Verification items for the finished model (mm, model axes). A direction names the side the tool comes from. Round coordinates to 2 decimals unless told otherwise and drop trailing zeros. Order: outer loops, then holes, each group sorted by start corner. A loop starts at its lowest first (then second) coordinate and runs counter-clockwise, first axis right, second up. Notation, with made-up numbers: M 40.25,-1.5 L 58.25,-1.5 A10 ccw 58.25,11.5 Z; hole C 65.25,59 d6. An arc over 180 degrees is marked long. Use one line per item in the form item = value. Start each with the question number.
Item 1: Thickness scan on probe 1 along X at (y, z) = (22, -120.65); probe 2 along Y at (x, z) = (1.5, -72.5); probe 3 along Z at (x, y) = (-11.5, -7) (3 decimals). Record the ranges inside material, lowest first. Write a range as [from, to].
Item 2: Cross-section at C-C on y = 0. Enter the section's corners in (x, z) (3 decimals), then the cut area to 3 significant figures.
Item 3: Cross-section at B-B on z = -120.65. Enter the section's corners in (x, y), then the cut area to 3 significant figures.
Item 4: Cross-section at A-A on x = -12.7. Enter the section's corners in (y, z) (3 decimals), then the cut area to 3 significant figures.
Item 5: Go/stop test with flat-tipped pins: pin 1 Ø3 at (x, y) = (-15.88, 21.82) entering from +Z; pin 2 Ø2.5 at (x, y) = (9.19, 9.19) entering from +Z (3 decimals); pin 3 Ø12 at (x, y) = (-14, 0.5) entering from -Z; pin 4 Ø2 at (x, z) = (10.5, -63.5) entering from -Y. Record where each tip stops, or that it passes through.
Item 6: Release check for a two-part mould opening along Z. For faces 4 (the cylindrical face through (12.881, 21.863, -119.273)), 5 (the cylindrical face through (12.881, 21.863, -20.848)), 6 (the cylindrical face through (-14.91, 23.32, 1.57)), 7 (the flat face through (0, 11, 3.175)) record: +Z half, -Z half, draft (parallel to the pull), parting line (faces both ways), or undercut.
Item 7: Cross-section at D-D on x = 0. Enter the section's corners in (y, z) (3 decimals), then the cut area to 3 significant figures.
Item 8: Tool access check on faces 1 (the cylindrical face through (-0.23, 23.59, 1.57)), 2 (the flat face through (0, 24.994, -61)), 3 (the flat face through (-0.3, 10.2, 0)). Record the directions out of +Z, -Z, +X, -X, +Y, -Y that give a thin tool (end or side, any length) a straight path to the whole face; none if there is none.
from build123d import *

# Parameters (mm, degrees)
SKETCH1_W           = 38.1
SKETCH1_H           = 37.6936
SKETCH1_R           = 10
SKETCH1_R_2         = 1.5
SKETCH1_R_3         = 1.7859375
BOSS_EXTRUDE1_DEPTH = 3.175
SKETCH2_W           = 38.1
SKETCH2_H           = 6.35
BOSS_EXTRUDE2_DEPTH = 127
CUT_EXTRUDE1_REACH  = 135.838
SKETCH3_R           = 1.3890625


with BuildPart() as part:
    # Sketch1 → Boss-Extrude1 (new body)
    with BuildSketch(Plane.XY):
        with Locations((0, 6.1468)):
            Rectangle(SKETCH1_W, SKETCH1_H)
        Circle(SKETCH1_R, mode=Mode.SUBTRACT)
        with Locations((-9.192388155, 9.192388155)):
            Circle(SKETCH1_R_2, mode=Mode.SUBTRACT)
        with Locations((9.192388155, 9.192388155)):
            Circle(SKETCH1_R_2, mode=Mode.SUBTRACT)
        with Locations((9.192388155, -9.192388155)):
            Circle(SKETCH1_R_2, mode=Mode.SUBTRACT)
        with Locations((-9.192388155, -9.192388155)):
            Circle(SKETCH1_R_2, mode=Mode.SUBTRACT)
        with Locations((15.875, 21.8186)):
            Circle(SKETCH1_R_3, mode=Mode.SUBTRACT)
        with Locations((0, 21.8186)):
            Circle(SKETCH1_R_3, mode=Mode.SUBTRACT)
        with Locations((-15.875, 21.8186)):
            Circle(SKETCH1_R_3, mode=Mode.SUBTRACT)
    extrude(amount=BOSS_EXTRUDE1_DEPTH)

    # Sketch2 → Boss-Extrude2 (add)
    with BuildSketch(Plane(origin=(0, 0, 0), x_dir=(-1, 0, 0), z_dir=(0, 0, -1))):
        with Locations((0, 21.8186)):
            Rectangle(SKETCH2_W, SKETCH2_H)
    extrude(amount=BOSS_EXTRUDE2_DEPTH)

    # Sketch3 → Cut-Extrude1 (cut, up to next)
    with BuildSketch(Plane(origin=(0, 24.9936, 0), x_dir=(1, 0, 0), z_dir=(0, 1, 0)), mode=Mode.PRIVATE) as cut_extrude1_sk1:
        with Locations(Location((-12.7, 120.65, 0), (0, 0, 180))):
            Circle(SKETCH3_R)
    cut_extrude1_tool1 = extrude(cut_extrude1_sk1.sketch, amount=-CUT_EXTRUDE1_REACH, mode=Mode.PRIVATE) & part.part
    # Sketch3 → Cut-Extrude1 (cut, up to next)
    with BuildSketch(Plane(origin=(0, 24.9936, 0), x_dir=(1, 0, 0), z_dir=(0, 1, 0)), mode=Mode.PRIVATE) as cut_extrude1_sk2:
        with Locations(Location((12.7, 120.65, 0), (0, 0, 180))):
            Circle(SKETCH3_R)
    cut_extrude1_tool2 = extrude(cut_extrude1_sk2.sketch, amount=-CUT_EXTRUDE1_REACH, mode=Mode.PRIVATE) & part.part
    # Sketch3 → Cut-Extrude1 (cut, up to next)
    with BuildSketch(Plane(origin=(0, 24.9936, 0), x_dir=(1, 0, 0), z_dir=(0, 1, 0)), mode=Mode.PRIVATE) as cut_extrude1_sk3:
        with Locations(Location((-12.7, 22.225, 0), (0, 0, 180))):
            Circle(SKETCH3_R)
    cut_extrude1_tool3 = extrude(cut_extrude1_sk3.sketch, amount=-CUT_EXTRUDE1_REACH, mode=Mode.PRIVATE) & part.part
    # Sketch3 → Cut-Extrude1 (cut, up to next)
    with BuildSketch(Plane(origin=(0, 24.9936, 0), x_dir=(1, 0, 0), z_dir=(0, 1, 0)), mode=Mode.PRIVATE) as cut_extrude1_sk4:
        with Locations(Location((12.7, 22.225, 0), (0, 0, 180))):
            Circle(SKETCH3_R)
    cut_extrude1_tool4 = extrude(cut_extrude1_sk4.sketch, amount=-CUT_EXTRUDE1_REACH, mode=Mode.PRIVATE) & part.part
    add(cut_extrude1_tool1.solids().sort_by_distance((-12.7, 24.9936, -120.65))[0], mode=Mode.SUBTRACT)
    add(cut_extrude1_tool2.solids().sort_by_distance((12.7, 24.9936, -120.65))[0], mode=Mode.SUBTRACT)
    add(cut_extrude1_tool3.solids().sort_by_distance((-12.7, 24.9936, -22.225))[0], mode=Mode.SUBTRACT)
    add(cut_extrude1_tool4.solids().sort_by_distance((12.7, 24.9936, -22.225))[0], mode=Mode.SUBTRACT)


solid = part.part
Output values:
q1.probe_1 = [-19.05, -14.09], [-11.31, 11.31], [14.09, 19.05]
q1.probe_2 = [18.64, 24.99]
q1.probe_3 = [0, 3.175]
q2.outline = M -19.05,0 L -10,0 L -10,3.175 L -19.05,3.175 Z; M 10,0 L 19.05,0 L 19.05,3.175 L 10,3.175 Z
q2.area = 57.5 mm2
q3.outline = M -19.05,18.64 L -14.09,18.64 L -14.09,24.99 L -19.05,24.99 Z; M -11.31,18.64 L 11.31,18.64 L 11.31,24.99 L -11.31,24.99 Z; M 14.09,18.64 L 19.05,18.64 L 19.05,24.99 L 14.09,24.99 Z
q3.area = 207 mm2
q4.outline = M -12.7,0 L 18.644,0 L 18.644,-20.836 L 24.994,-20.836 L 24.994,3.175 L -12.7,3.175 Z; M 18.644,-127 L 24.994,-127 L 24.994,-122.039 L 18.644,-122.039 Z; M 18.644,-119.261 L 24.994,-119.261 L 24.994,-23.614 L 18.644,-23.614 Z
q4.area = 891 mm2
q5.pin_1 = 0
q5.pin_2 = through
q5.pin_3 = 0
q5.pin_4 = 18.64
q6.face_4 = undercut
q6.face_5 = undercut
q6.face_6 = draft
q6.face_7 = +Z half
q7.outline = M -12.7,0 L -10,0 L -10,3.175 L -12.7,3.175 Z; M 10,0 L 18.644,0 L 18.644,-127 L 24.994,-127 L 24.994,3.175 L 23.605,3.175 L 23.605,0 L 20.033,0 L 20.033,3.175 L 10,3.175 Z
q7.area = 851 mm2
q8.face_1 = +Z
q8.face_2 = +Z, -Z, +X, -X, +Y
q8.face_3 = -Z, +X, -X, -Y
